from build123d import *

# Parameters (mm, degrees)
F1_R     = 4.625
F1_R_2   = 2.425
F2_DEPTH = 2
F3_START = 1.5
F3_DEPTH = 0.5
F4_START = 2
F4_DEPTH = 36
F5_SIZE2 = 2
F5_SIZE  = 1.25
F6_R     = 0.25


# Not quite as in the source:
# - a feature names something its author has since deleted; it is built from what else it names


with BuildPart() as f2:
    # F1 (on Top) → F2 (new body)
    with BuildSketch(Plane.XY):
        Circle(F1_R)
        Circle(F1_R_2, mode=Mode.SUBTRACT)
        Circle(F1_R_2)
        Polygon((-0.9381941874, -1.625), (-1.8763883749, 0), (-0.9381941874, 1.625), (0.9381941874, 1.625), (1.8763883749, 0), (0.9381941874, -1.625), align=None, mode=Mode.SUBTRACT)
    extrude(amount=F2_DEPTH)

    # F1 (on Top) → F3 (join)
    with BuildSketch(Plane.XY.offset(F3_START)):
        Polygon((-0.9381941874, 1.625), (-1.8763883749, 0), (-0.9381941874, -1.625), (0.9381941874, -1.625), (1.8763883749, 0), (0.9381941874, 1.625), align=None)
    extrude(amount=F3_DEPTH)

    # F1 (on Top) → F4 (join)
    with BuildSketch(Plane.XY.offset(F4_START)):
        Circle(F1_R_2)
        Polygon((-0.9381941874, -1.625), (-1.8763883749, 0), (-0.9381941874, 1.625), (0.9381941874, 1.625), (1.8763883749, 0), (0.9381941874, -1.625), align=None, mode=Mode.SUBTRACT)
        Polygon((-0.9381941874, 1.625), (-1.8763883749, 0), (-0.9381941874, -1.625), (0.9381941874, -1.625), (1.8763883749, 0), (0.9381941874, 1.625), align=None)
    extrude(amount=F4_DEPTH)

    # F5
    f5_edges = [f2.edges().sort_by_distance(p)[0] for p in [
        (-4.625, 0, 0),
    ]]
    f5_side = f2.faces().sort_by_distance((-4.625, 0, 1))[0]
    chamfer(f5_edges, length=F5_SIZE, length2=F5_SIZE2, reference=f5_side)

    # F6
    f6_edges = [f2.edges().sort_by_distance(p)[0] for p in [
        (-4.625, 0, 2),
        (-2.425, 0, 2),
        (-2.625, 0, 0),
        (-4.625, 0, 1.25),
    ]]
    fillet(f6_edges, radius=F6_R)


solid = f2.part
Can you work these out from the model? Positions are in its coordinate system, mm. A direction names the side the tool comes from. Give positions to 0.01 mm unless a question says otherwise; leave off trailing zeros. Order: outer loops, then holes, each group sorted by start corner. A loop starts at its lowest first (then second) coordinate and runs counter-clockwise, first axis right, second up. Notation, with made-up numbers: M 20,56.5 L 47,56.5 A15 ccw 47,62.5 Z; hole C 44.5,-10.5 d1. An arc over 180 degrees is marked long. One line per question, with ' | ' between items.
Item 1: Suppose I cut it at A-A, the plane z = 17. Write out the boundary of the cut face in (x, y) (3 decimals).
Answer block:
outline: C 0,0 d4.85
Item 2: Please list where these lines run through material, in increasing order: L1, parallel to Z at x = -0.75, y = -0.5; L2, parallel to Y at x = -0.75, z = 18.5; L3, parallel to Z at x = 4.25, y = 1.5.
Answer block:
L1: z = 1.5 to 38 | L2: y = -2.31 to 2.31 | L3: z = 1.18 to 1.96
Item 3: We'd pull the mould along X, two halves only. Please class faces 4 (the face through (2.313, 0.728, 19.875)), 5 (the face through (-1.414, 0.801, 0.74)), 6 (the face through (0, -2, 0)): released by +X, released by -X, zero draft, split by the parting line, or undercut.
Answer block:
face 4: split by the parting line | face 5: undercut | face 6: zero draft
Item 4: I'm going to push flat-ended pins straight in: pin 1 Ø3 at (x, y) = (-2.5, 3.5) entering from -Z; pin 2 Ø5 at (y, z) = (-1, 33) entering from +X (3 decimals); pin 3 Ø0.8 at (x, z) = (0.5, 1) entering from +Y. Where does each tip first touch, or does it pass through?
Answer block:
pin 1: stops at z = 0.11 | pin 2: stops at x = 2.425 | pin 3: stops at y = 4.61
Item 5: For faces 1 (the face through (0, -1.625, 1)), 2 (the face through (-2, -2, 2)), 3 (the face through (-1.003, -4.515, 1.567)), which set-ups out of +Z, -Z, +X, -X, +Y, -Y let a thin tool reach every point of the face, with its end or its side?
Answer block:
face 1: -Z | face 2: +Z | face 3: +Z, -Z
